Read the model definition and answer for the solid it produces. Units are mm, in the model's axes. A direction names the side the tool comes from. Coordinates: 2 decimals unless noted, no trailing zeros. Loops run counter-clockwise (first coordinate to the right, second up) from the corner with the lowest first, then second, coordinate; pieces in that order, holes last. Notation, with made-up numbers: (81.5, 52.25) - (98.5, 52.25) arc R16 cw to (98.5, 59.25) - close; hole circle Ø4 at (-35.5, 2). An arc over 180 degrees is marked (long way). Use one line per item in the form item = value.
from build123d import *

# Parameters (mm, degrees)
SALIENTE_EXTRUIR1_DEPTH = 35
CROQUIS4_R              = 2
CORTAR_EXTRUIR1_DEPTH   = 2
CROQUIS5_R              = 1.25
CORTAR_EXTRUIR2_DEPTH   = 57.632946618
CROQUIS6_W              = 12
CROQUIS6_H              = 8
CORTAR_EXTRUIR3_DEPTH   = 58.094315502
CROQUIS7_R              = 2.4
CROQUIS7_R_2            = 1.6
SALIENTE_EXTRUIR3_DEPTH = 2
CROQUIS10_R             = 1.6
CORTAR_EXTRUIR6_DEPTH   = 58.094315502
REDONDEO1_R             = 3


with BuildPart() as part:
    # Croquis3 → Saliente-Extruir1 (new body)
    with BuildSketch(Plane(origin=(0, 0, 0), x_dir=(0, 0, -1), z_dir=(1, 0, 0))):
        with BuildLine():
            Line((15.15, 26.240569735), (27.267552537, 26.240569735))
            Line((27.267552537, 26.240569735), (27.267552537, 42.842217067))
            Line((27.267552537, 42.842217067), (29.267552537, 42.842217067))
            Line((29.267552537, 42.842217067), (29.267552537, 7.842217067))
            ThreePointArc((29.267552537, 7.842217067), (24.038606211, 18.445471299), (15.15, 26.240569735))
        make_face()
    extrude(amount=SALIENTE_EXTRUIR1_DEPTH)

    # Croquis4 → Cortar-Extruir1 (cut)
    with BuildSketch(Plane(origin=(0, 0, -29.267552537), x_dir=(-1, 0, 0), z_dir=(0, 0, -1))):
        with Locations((-25, 19.842217067)):
            Circle(CROQUIS4_R)
        with Locations((-10, 19.842217067)):
            Circle(CROQUIS4_R)
    extrude(amount=-CORTAR_EXTRUIR1_DEPTH, mode=Mode.SUBTRACT)

    # Croquis5 → Cortar-Extruir2 (cut, through all)
    with BuildSketch(Plane(origin=(0, 0, -27.267552537), x_dir=(-1, 0, 0), z_dir=(0, 0, -1))):
        with Locations((-25, 19.842217067)):
            Circle(CROQUIS5_R)
        with Locations((-10, 19.842217067)):
            Circle(CROQUIS5_R)
    extrude(amount=-CORTAR_EXTRUIR2_DEPTH, mode=Mode.SUBTRACT)

    # Croquis6 → Cortar-Extruir3 (cut, through all)
    with BuildSketch(Plane(origin=(0, 0, -29.267552537), x_dir=(-1, 0, 0), z_dir=(0, 0, -1))):
        with Locations((-12.35, 11.842217067)):
            Rectangle(CROQUIS6_W, CROQUIS6_H)
    extrude(amount=-CORTAR_EXTRUIR3_DEPTH, mode=Mode.SUBTRACT)

    # Croquis7 → Saliente-Extruir3 (add)
    # profile 1 of 4: a face of its own
    with BuildSketch(Plane(origin=(0, 0, -29.267552537), x_dir=(-1, 0, 0), z_dir=(0, 0, -1))):
        with Locations(Location((-31.5, 39.492217067, 0), (0, 0, 180))):
            Circle(CROQUIS7_R)
        with Locations((-31.5, 39.492217067)):
            Circle(CROQUIS7_R_2, mode=Mode.SUBTRACT)
    # profile 2 of 4: a face of its own
    with BuildSketch(Plane(origin=(0, 0, -29.267552537), x_dir=(-1, 0, 0), z_dir=(0, 0, -1))):
        with Locations(Location((-3.5, 39.492217067, 0), (0, 0, 180))):
            Circle(CROQUIS7_R)
        with Locations((-3.5, 39.492217067)):
            Circle(CROQUIS7_R_2, mode=Mode.SUBTRACT)
    # profile 3 of 4: a face of its own
    with BuildSketch(Plane(origin=(0, 0, -29.267552537), x_dir=(-1, 0, 0), z_dir=(0, 0, -1))):
        with Locations(Location((-3.5, 11.492217067, 0), (0, 0, 180))):
            Circle(CROQUIS7_R)
        with Locations((-3.5, 11.492217067)):
            Circle(CROQUIS7_R_2, mode=Mode.SUBTRACT)
    # profile 4 of 4: a face of its own
    with BuildSketch(Plane(origin=(0, 0, -29.267552537), x_dir=(-1, 0, 0), z_dir=(0, 0, -1))):
        with Locations(Location((-31.5, 11.492217067, 0), (0, 0, 180))):
            Circle(CROQUIS7_R)
        with Locations((-31.5, 11.492217067)):
            Circle(CROQUIS7_R_2, mode=Mode.SUBTRACT)
    extrude(amount=SALIENTE_EXTRUIR3_DEPTH)

    # Croquis10 → Cortar-Extruir6 (cut, through all)
    with BuildSketch(Plane(origin=(0, 0, -29.267552537), x_dir=(-1, 0, 0), z_dir=(0, 0, -1))):
        with Locations((-31.5, 11.492217067)):
            Circle(CROQUIS10_R)
        with Locations((-3.5, 11.492217067)):
            Circle(CROQUIS10_R)
        with Locations((-3.5, 39.492217067)):
            Circle(CROQUIS10_R)
        with Locations((-31.5, 39.492217067)):
            Circle(CROQUIS10_R)
    extrude(amount=-CORTAR_EXTRUIR6_DEPTH, mode=Mode.SUBTRACT)

    # Redondeo1
    redondeo1_edges = [part.edges().sort_by_distance(p)[0] for p in [
        (35, 42.842217067, -28.267552537),
        (0, 42.842217067, -28.267552537),
    ]]
    fillet(redondeo1_edges, radius=REDONDEO1_R)


solid = part.part
Item 1: The part is cut by section A-A on x = 25. Give the vertices of the cut face in (y, z).
Results below:
outline = (7.84, -29.27) - (17.84, -29.27) - (17.84, -27.27) - (18.59, -27.27) - (18.59, -23.93) arc R30.3 cw to start; (21.09, -27.27) - (21.84, -27.27) - (21.84, -29.27) - (42.84, -29.27) - (42.84, -27.27) - (26.24, -27.27) - (26.24, -15.15) arc R30.3 cw to (21.09, -21.75) - close
Item 2: Which of the six approach directions +Z, -Z, +X, -X, +Y, -Y give full straight-line access (tool end or side, diameter ignored) to faces 4 (the flat face through (12, 15.842, -28)), 5 (the cylindrical face through (31.188, 37.113, -30.254)), 6 (the cylindrical face through (10.16, 21.08, -25.16))?
Results below:
face_4 = +Z, -Z, -Y
face_5 = -Z
face_6 = +Z, -Z
Item 3: The part is cut by section D-D on x = 31.5. Give the vertices of the cut face in (y, z).
Results below:
outline = (7.84, -29.27) - (9.09, -29.27) - (9.09, -31.27) - (9.89, -31.27) - (9.89, -28.64) arc R30.3 cw to start; (13.09, -31.27) - (13.89, -31.27) - (13.89, -29.27) - (37.09, -29.27) - (37.09, -31.27) - (37.89, -31.27) - (37.89, -27.27) - (26.24, -27.27) - (26.24, -15.15) arc R30.3 cw to (13.09, -27.33) - close; (41.09, -31.27) - (41.89, -31.27) - (41.89, -29.27) - (42.84, -29.27) - (42.84, -27.27) - (41.09, -27.27) - close
Item 4: Each of these flat-tipped pins is pushed along its axis until it touches: P1, Ø3, axis at x = 17, z = -23, coming from the +Y side; P2, Ø3, axis at x = 31.5, y = 11.49, coming from the -Z side; P3, Ø1.5, axis at x = 19, y = 11.5, coming from the -Z side; P4, Ø4.5, axis at x = 25, y = 19.84, coming from the +Z side. Where does it stop, or does it pass through?
Results below:
P1 = 26.24
P2 = through
P3 = -29.27
P4 = -20.74
Item 5: The part is cut by section B-B on z = -25. Give the vertices of the cut face in (x, y).
Results below:
outline = (0, 17.12) - (35, 17.12) - (35, 26.24) - (0, 26.24) - close; hole circle Ø2.5 at (10, 19.84); hole circle Ø2.5 at (25, 19.84)
Item 6: The part is cut by section C-C on y = 28.5. Give the vertices of the cut face in (x, z), plus the area to 3 significant figures.
Results below:
outline = (0, -29.27) - (35, -29.27) - (35, -27.27) - (0, -27.27) - close
area = 70.0 mm²
Item 7: For a pull along X with two mould halves and no side action, classify faces 1 (the cylindrical face through (3.188, 37.113, -30.254)), 2 (the flat face through (17, 26.241, -21)), 3 (the flat face through (0, 24, -26)) as +X half, -X half, draft (parallel to the pull), parting line (faces both ways), or undercut.
Results below:
face_1 = undercut
face_2 = draft
face_3 = -X half
Item 8: Find the intervals of material crossed by L1, parallel to Y at x = 31.5, z = -30.5; L2, parallel to X at y = 20, z = -28; L3, parallel to Y at x = 4, z = -29.5, in increasing order.
Results below:
L1 = 9.09 to 9.89, 13.09 to 13.89, 37.09 to 37.89, 41.09 to 41.89
L2 = 0 to 8.01, 11.99 to 23.01, 26.99 to 35
L3 = 9.14 to 9.97, 13.01 to 13.84, 37.14 to 37.97, 41.01 to 41.84
